Verification items for the finished model (mm, model axes). Round coordinates to 2 decimals unless told otherwise and drop trailing zeros. Loops run counter-clockwise (first coordinate to the right, second up) from the corner with the lowest first, then second, coordinate; pieces in that order, holes last. Notation, with made-up numbers: M 23.25,67.25 L 63.25,67.25 A24 ccw 63.25,101.25 Z; hole C -11,52 d6. An arc over 180 degrees is marked long. One line per item, written item: value.
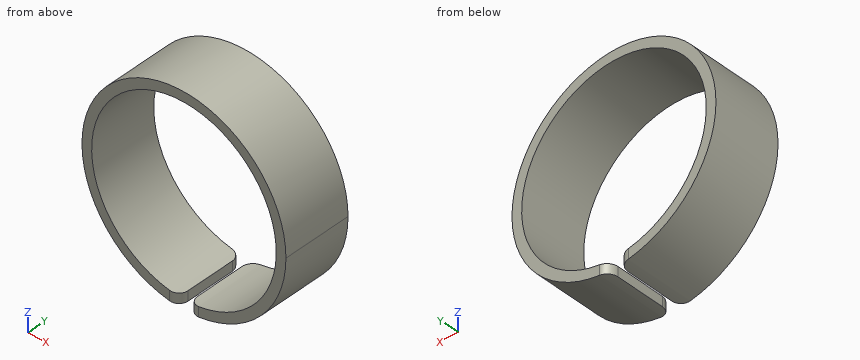
from build123d import *

# Parameters (mm, degrees)
SKETCH3_R               = 10.52
SKETCH3_R_2             = 9.52
EXTRUDE_THIN1_DEPTH     = 3.5
SKETCH4_W               = 1
SKETCH4_H               = 1000
CUT_EXTRUDE1_DEPTH      = 4.5
CUT_EXTRUDE1_DEPTH_BACK = 4.5
FILLET1_R               = 1


with BuildPart() as part:
    # Sketch3 → Extrude-Thin1 (new body, symmetric)
    with BuildSketch(Plane(origin=(0, 0, 0), x_dir=(1, 0, 0), z_dir=(0, 1, 0))):
        Circle(SKETCH3_R)
        Circle(SKETCH3_R_2, mode=Mode.SUBTRACT)
    extrude(amount=EXTRUDE_THIN1_DEPTH, both=True)

    # Sketch4 → Cut-Extrude1 (cut, two sides)
    with BuildSketch(Plane(origin=(0, 0, 0), x_dir=(1, 0, 0), z_dir=(0, 1, 0))) as cut_extrude1_sk:
        with Locations((0, 500)):
            Rectangle(SKETCH4_W, SKETCH4_H)
    extrude(amount=CUT_EXTRUDE1_DEPTH, mode=Mode.SUBTRACT)
    extrude(cut_extrude1_sk.sketch, amount=-CUT_EXTRUDE1_DEPTH_BACK, mode=Mode.SUBTRACT)

    # Fillet1
    fillet1_edges = [part.edges().sort_by_distance(p)[0] for p in [
        (0.5, -3.5, -10.007485917),
        (-0.5, -3.5, -10.007485917),
        (0.5, 3.5, -10.007485917),
        (-0.5, 3.5, -10.007485917),
    ]]
    fillet(fillet1_edges, radius=FILLET1_R)


solid = part.part
(1) Sectioned sample at A-A on z = -4.25. Enter the section's corners in (x, y), and give its area (3 significant figures).
Completed:
outline: M -9.62,-3.5 L -8.52,-3.5 L -8.52,3.5 L -9.62,3.5 Z; M 8.52,-3.5 L 9.62,-3.5 L 9.62,3.5 L 8.52,3.5 Z
area: 15.5 mm^2
(2) Thickness scan on L1, parallel to X at y = 2, z = 0; L2, parallel to Z at x = 0, y = 0; L3, parallel to Z at x = 2.75, y = 2.5. Record the ranges inside material, lowest first. Write a range as from..to.
Completed:
L1: x = -10.52..-9.52, 9.52..10.52
L2: z = 9.52..10.52
L3: z = -10.15..-9.11, 9.11..10.15
(3) Sectioned sample at B-B on x = 9. Enter the section's corners in (y, z).
Completed:
outline: M -3.5,-5.45 L 3.5,-5.45 L 3.5,-3.1 L -3.5,-3.1 Z; M -3.5,3.1 L 3.5,3.1 L 3.5,5.45 L -3.5,5.45 Z
(4) Sectioned sample at C-C on y = -1.5. Enter the section's corners in (x, z).
Completed:
outline: M -0.5,-10.51 L -0.5,-9.51 A9.52 cw long 0.5,-9.51 L 0.5,-10.51 A10.52 ccw long Z
(5) Depth check by flat-ended pin: pin 1 Ø3 at (y, z) = (-2, -7) entering from +X; pin 2 Ø0.8 at (y, z) = (1, -10) entering from +X; pin 3 Ø8 at (x, z) = (1, -8) entering from +Y; pin 4 Ø0.8 at (y, z) = (0, -10) entering from -X. Enter the tip coordinate at first touch or a pass-through.
Completed:
pin 1: stops at x = 8.97
pin 2: stops at x = 4.3
pin 3: stops at y = 3.5
pin 4: stops at x = -4.3
(6) Sectioned sample at D-D on x = 0. Enter the section's corners in (y, z), and give its area (3 significant figures).
Completed:
outline: M -3.5,9.52 L 3.5,9.52 L 3.5,10.52 L -3.5,10.52 Z
area: 7.00 mm^2
